Can you work these out from the model? Positions are in its coordinate system, mm. A direction names the side the tool comes from. Coordinates: 2 decimals unless noted, no trailing zeros. Write each loop counter-clockwise with the first axis right and the second up, starting at its lowest first coordinate (ties: lowest second). Pieces come first, ordered by that corner, then holes. Notation, with made-up numbers: (81, 60.5) -> (88, 60.5) arc R4 ccw to (88, 66.5) -> close; hole circle Ø1 at (-22, 35). An arc over 180 degrees is marked (long way). Use one line per item in the form item = value.
```python
from build123d import *

# Parameters (mm, degrees)
F0_R     = 5.5
F0_R_2   = 4
F1_DEPTH = 12
F2_D     = 3
F3_R     = 2.5
F3_R_2   = 1.5
F4_DEPTH = 12
F6_DEPTH = 5


# Not quite as in the source:
# - a feature of the source that left no trace in its solid (it failed there, or was rolled back) is left out


with BuildPart() as f1:
    # F0 (on Top) → F1 (new body)
    with BuildSketch(Plane.XY):
        with BuildLine():
            Line((13, 12), (-13, 12))
            ThreePointArc((-13, 12), (-16.5355339059, 10.5355339059), (-18, 7))
            Line((-18, 7), (-18, -7))
            ThreePointArc((-18, -7), (-16.5355339059, -10.5355339059), (-13, -12))
            Line((-13, -12), (13, -12))
            ThreePointArc((13, -12), (16.5355339059, -10.5355339059), (18, -7))
            Line((18, -7), (18, 7))
            ThreePointArc((18, 7), (16.5355339059, 10.5355339059), (13, 12))
        make_face()
        Circle(F0_R, mode=Mode.SUBTRACT)
        Circle(F0_R)
        Circle(F0_R_2, mode=Mode.SUBTRACT)
        Circle(F0_R_2)
    extrude(amount=F1_DEPTH)

    # F2 (through all)
    with Locations(Plane(origin=(0, 0, 0), x_dir=(1, 0, 0), z_dir=(0, 0, -1))):
        with Locations((15, 0), (0, 9), (0, -9), (-15, 0)):
            Hole(F2_D / 2)

    # F3 (on face) → F4 (join, through all)
    with BuildSketch(Plane.XY):
        with Locations((0, 9)):
            Circle(F3_R)
        with Locations((0, 9)):
            Circle(F3_R_2, mode=Mode.SUBTRACT)
        with Locations((0, -9)):
            Circle(F3_R)
        with Locations((0, -9)):
            Circle(F3_R_2, mode=Mode.SUBTRACT)
    extrude(amount=F4_DEPTH)

    # F0 (on Top) → F6 (join)
    with BuildSketch(Plane.XY):
        Circle(F0_R)
        Circle(F0_R_2, mode=Mode.SUBTRACT)
    extrude(amount=-F6_DEPTH)


solid = f1.part
```
Q1. Suppose I cut it at B-B (y = 0). Write out the boundary of the cut face in (x, z).
Return value:
outline = (-18, 0) -> (-16.5, 0) -> (-16.5, 12) -> (-18, 12) -> close; (-13.5, 0) -> (-5.5, 0) -> (-5.5, -5) -> (-4, -5) -> (-4, 0) -> (4, 0) -> (4, -5) -> (5.5, -5) -> (5.5, 0) -> (13.5, 0) -> (13.5, 12) -> (-13.5, 12) -> close; (16.5, 0) -> (18, 0) -> (18, 12) -> (16.5, 12) -> close
Q2. Suppose I cut it at D-D (x = -14). Write out the boundary of the cut face in (y, z).
Return value:
outline = (-11.9, 0) -> (-1.12, 0) -> (-1.12, 12) -> (-11.9, 12) -> close; (1.12, 0) -> (11.9, 0) -> (11.9, 12) -> (1.12, 12) -> close
Q3. Suppose I cut it at C-C (z = 6.75). Write out the boundary of the cut face in (x, y), then the cut area to 3 significant figures.
Return value:
outline = (-18, -7) arc R5 ccw to (-13, -12) -> (13, -12) arc R5 ccw to (18, -7) -> (18, 7) arc R5 ccw to (13, 12) -> (-13, 12) arc R5 ccw to (-18, 7) -> close; hole circle Ø3 at (-15, 0); hole circle Ø3 at (0, -9); hole circle Ø3 at (0, 9); hole circle Ø3 at (15, 0)
area = 814 mm2
Q4. Will this pin go through, and if not, where does the flat tip stop? pin 1 (8 mm diameter, centred on x = -12, y = -2, fed in from -Z).
Return value:
pin_1 = 0
Q5. Thinking about a two-plate mould opening in X: for faces 3 (the flat face through (18, 0, 6)), 4 (the cylindrical face through (-13.5, -0.07, 6.08)), 5 (the flat face through (0, 6, 0)), 6 (the cylindrical face through (0.325, -7.536, 6.084)), which applies, released by +X, released by -X, zero draft, split by the parting line, or undercut?
Return value:
face_3 = released by +X
face_4 = undercut
face_5 = zero draft
face_6 = undercut
Q6. If I drill on line 1 (Y direction, x = 0, z = 7.5); line 2 (Y direction, x = 0, z = -1.9); line 3 (X direction, y = 1.25, z = 1.5), over which ranges is the centre line in solid material (lowest first)? Write a range as from..to.
Return value:
line_1 = -12..-10.5, -7.5..7.5, 10.5..12
line_2 = -5.5..-4, 4..5.5
line_3 = -18..-15.83, -14.17..14.17, 15.83..18
Q7. For faces 1 (the cylindrical face through (16.5, -0.07, 6.08)), 2 (the cylindrical face through (-0.867, -3.905, -2.465)), which set-ups out of +Z, -Z, +X, -X, +Y, -Y let a thin tool reach every point of the face, with its end or its side?
Return value:
face_1 = +Z, -Z
face_2 = -Z
Q8. Suppose I cut it at A-A (x = 0). Write out the boundary of the cut face in (y, z), then the cut area to 3 significant figures.
Return value:
outline = (-12, 0) -> (-10.5, 0) -> (-10.5, 12) -> (-12, 12) -> close; (-7.5, 0) -> (-5.5, 0) -> (-5.5, -5) -> (-4, -5) -> (-4, 0) -> (4, 0) -> (4, -5) -> (5.5, -5) -> (5.5, 0) -> (7.5, 0) -> (7.5, 12) -> (-7.5, 12) -> close; (10.5, 0) -> (12, 0) -> (12, 12) -> (10.5, 12) -> close
area = 231 mm2
